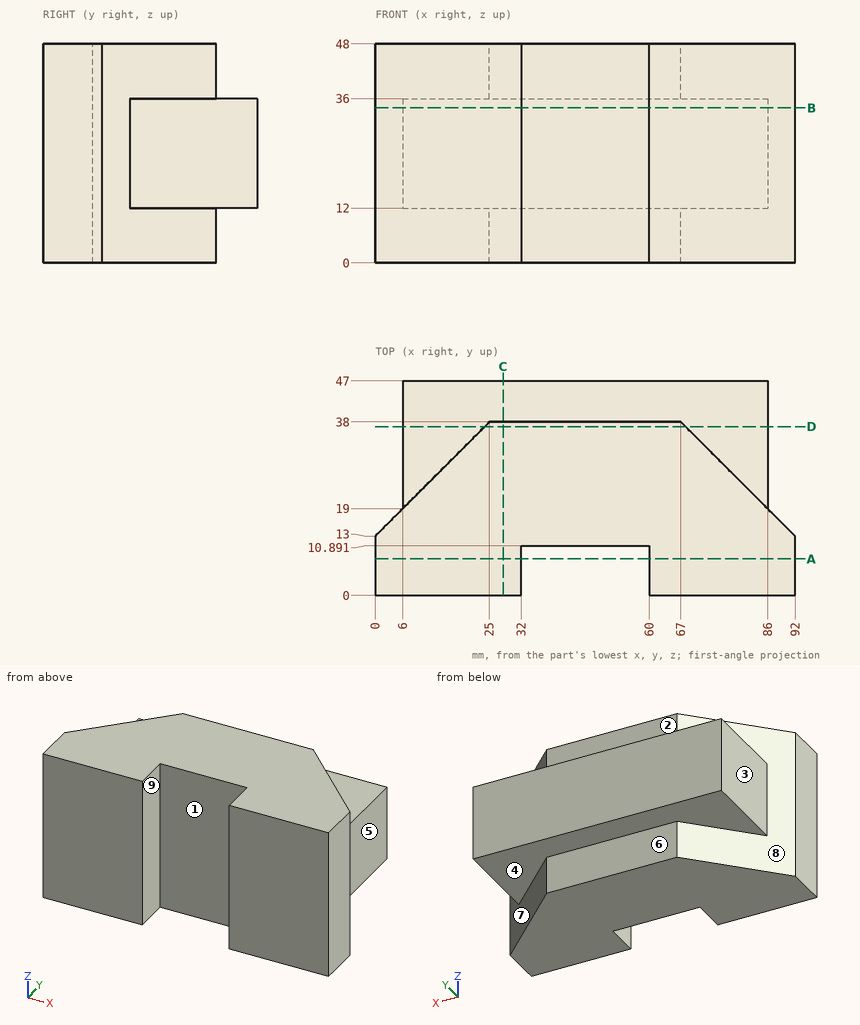
Drawing for the job (mm, zero at the part's lowest x, y, z). A direction names the side the tool comes from. Round coordinates to 2 decimals unless told otherwise and drop trailing zeros. Loops run counter-clockwise (first coordinate to the right, second up) from the corner with the lowest first, then second, coordinate; pieces in that order, holes last. Notation, with made-up numbers: (72.5, 62.25) - (126.5, 62.25) arc R31 ccw to (126.5, 98.25) - close; hole circle Ø10 at (84.5, 48). An arc over 180 degrees is marked (long way). Return JSON: item names as keys, results as strings. Group by question number.
Q1. Two-plate mould, pull along X, no slides. Class the marked faces 6, 7, 8 and 9: +X half, -X half, draft (parallel to the pull), parting line (faces both ways), or undercut.
Q2. Band-saw the part on B-B on z = 34. Give the cut face in (x, y), plus the area to 3 significant figures.
Q3. Tool access for the marked faces 1, 2, 3, 4 and 5: list every direction of +Z, -Z, +X, -X, +Y, -Y with a clear straight run to the whole face (end or side of a thin tool).
Q4. Drill centre lines: line 1 along X through (y, z) = (10, 24); line 2 along Z through (x, y) = (84.5, 24); line 3 along Y through (x, z) = (52, 20.5). Where is each one in solid material? Low to high. Write a range as [from, to].
Q5. Band-saw the part on A-A on y = 8. Give the cut face in (x, z), plus the area to 3 significant figures.
Q6. Band-saw the part on D-D on y = 37. Give the cut face in (x, z), plus the area to 3 significant figures.
Q7. Band-saw the part on C-C on x = 28. Give the cut face in (y, z), plus the area to 3 significant figures.
Q8. Flat gauge pins, fed straight in: pin 1 Ø2 at (x, y) = (48, 39.5) entering from +Z; pin 2 Ø1 at (y, z) = (14, 10.5) entering from -X; pin 3 Ø8.5 at (x, z) = (39.5, 21) entering from -Y. Where does each tip first touch, or does it go through?
Solutions:
{
 "1": {"face 6": "draft", "face 7": "+X half", "face 8": "-X half", "face 9": "undercut"},
 "2": {"outline": "(0, 0) - (32, 0) - (32, 10.89) - (60, 10.89) - (60, 0) - (92, 0) - (92, 13) - (86, 19) - (86, 47) - (6, 47) - (6, 19) - (0, 13) - close", "area": "3,650 mm^2"},
 "3": {"face 1": "+Z, -Z, -Y", "face 2": "+Z, +X, -X, +Y", "face 3": "+Z, -Z, -X, +Y", "face 4": "-Z, +Y", "face 5": "+Z, -Z, +X, +Y"},
 "4": {"line 1": "x = [0, 32], [60, 92]", "line 2": "z = [12, 36]", "line 3": "y = [10.89, 47]"},
 "5": {"outline": "(0, 0) - (32, 0) - (32, 48) - (0, 48) - close; (60, 0) - (92, 0) - (92, 48) - (60, 48) - close", "area": "3,070 mm^2"},
 "6": {"outline": "(6, 12) - (24, 12) - (24, 0) - (68, 0) - (68, 12) - (86, 12) - (86, 36) - (68, 36) - (68, 48) - (24, 48) - (24, 36) - (6, 36) - close", "area": "2,980 mm^2"},
 "7": {"outline": "(0, 0) - (38, 0) - (38, 12) - (47, 12) - (47, 36) - (38, 36) - (38, 48) - (0, 48) - close", "area": "2,040 mm^2"},
 "8": {"pin 1": "stops at z = 36", "pin 2": "stops at x = 0.5", "pin 3": "stops at y = 10.89"}
}
